Check sheet for the modelled part. Datum: model origin and axes. Units: mm. A direction names the side the tool comes from. Give positions to 0.01 mm unless a question says otherwise; leave off trailing zeros. Loops run counter-clockwise (first coordinate to the right, second up) from the corner with the lowest first, then second, coordinate; pieces in that order, holes last. Notation, with made-up numbers: M 7,20.5 L 44,20.5 A12 cw 44,35.5 Z; hole C 17,82 d4. An arc over 180 degrees is marked long. Use one line per item in the form item = value.
from build123d import *

# Parameters (mm, degrees)
SKETCH2_W           = 82.55
SKETCH2_H           = 38.1
BOSS_EXTRUDE1_DEPTH = 2.54
SKETCH3_W           = 71.12
SKETCH3_H           = 25.4
BOSS_EXTRUDE2_DEPTH = 5.08
SKETCH4_W           = 68.58
SKETCH4_H           = 22.86
CUT_EXTRUDE1_DEPTH  = 1.27
CUT_EXTRUDE1_DRAFT  = -18
SKETCH5_R           = 2.54
CUT_EXTRUDE2_DEPTH  = 2.54


with BuildPart() as part:
    # Sketch2 → Boss-Extrude1 (new body)
    with BuildSketch(Plane(origin=(0, 0, 0), x_dir=(1, 0, 0), z_dir=(0, 1, 0))):
        Rectangle(SKETCH2_W, SKETCH2_H)
    extrude(amount=BOSS_EXTRUDE1_DEPTH)

    # Sketch3 → Boss-Extrude2 (add)
    with BuildSketch(Plane(origin=(0, 2.54, 0), x_dir=(1, 0, 0), z_dir=(0, 1, 0))):
        Rectangle(SKETCH3_W, SKETCH3_H)
    extrude(amount=BOSS_EXTRUDE2_DEPTH)


with BuildPart() as cut_extrude1_tool:
    # Sketch4 → Cut-Extrude1 (with draft: the straight prism first)
    with BuildSketch(Plane(origin=(0, 7.62, 0), x_dir=(1, 0, 0), z_dir=(0, 1, 0))):
        Rectangle(SKETCH4_W, SKETCH4_H)
    extrude(amount=-CUT_EXTRUDE1_DEPTH)
    # Cut-Extrude1: the draft: its side faces are tilted about the plane it starts from
    cut_extrude1_sides = [cut_extrude1_tool.faces().sort_by_distance(p)[0] for p in [
        (-34.29, 6.985, 0),
        (0, 6.985, 11.43),
        (34.29, 6.985, 0),
        (0, 6.985, -11.43),
    ]]
    draft(cut_extrude1_sides, Plane(origin=(0, 7.62, 0), x_dir=(1, 0, 0), z_dir=(0, 1, 0)), CUT_EXTRUDE1_DRAFT)


with BuildPart() as part_1:
    add(part.part)

    # Cut-Extrude1: cut by cut_extrude1_tool
    add(cut_extrude1_tool.part, mode=Mode.SUBTRACT)

    # Sketch5 → Cut-Extrude2 (cut)
    with BuildSketch(Plane(origin=(0, 2.54, 0), x_dir=(1, 0, 0), z_dir=(0, 1, 0))):
        with Locations(Location((-37.465, 15.875, 0), (0, 0, 270))):
            Circle(SKETCH5_R)
        with Locations(Location((-37.465, -15.875, 0), (0, 0, 270))):
            Circle(SKETCH5_R)
        with Locations(Location((37.465, -15.875, 0), (0, 0, 270))):
            Circle(SKETCH5_R)
        with Locations(Location((37.465, 15.875, 0), (0, 0, 270))):
            Circle(SKETCH5_R)
    extrude(amount=-CUT_EXTRUDE2_DEPTH, mode=Mode.SUBTRACT)


solid = part_1.part
1) Section check C-C (z = 17.5). Record the cut outline in (x, y) (3 decimals), then the cut area to 3 significant figures.
Evaluation:
outline = M -41.275,0 L -39.417,0 L -39.417,2.54 L -41.275,2.54 Z; M -35.513,0 L 35.513,0 L 35.513,2.54 L -35.513,2.54 Z; M 39.417,0 L 41.275,0 L 41.275,2.54 L 39.417,2.54 Z
area = 190 mm^2
2) Section check B-B (x = 29). Record the cut outline in (y, z).
Evaluation:
outline = M 0,-19.05 L 2.54,-19.05 L 2.54,-12.7 L 7.62,-12.7 L 7.62,-11.43 L 6.35,-11.02 L 6.35,11.02 L 7.62,11.43 L 7.62,12.7 L 2.54,12.7 L 2.54,19.05 L 0,19.05 Z
3) Section check A-A (z = -1). Record the cut outline in (x, y) (3 decimals).
Evaluation:
outline = M -41.275,0 L 41.275,0 L 41.275,2.54 L 35.56,2.54 L 35.56,7.62 L 34.29,7.62 L 33.877,6.35 L -33.877,6.35 L -34.29,7.62 L -35.56,7.62 L -35.56,2.54 L -41.275,2.54 Z
4) Set-up check for faces 4 (the face through (0, 5, 12.7)), 5 (the face through (0, 6.35, 0)), 6 (the face through (0, 5, -12.7)), 7 (the face through (-35.56, 5, 0)), 8 (the face through (35.56, 5, 0)): record each of +Z, -Z, +X, -X, +Y, -Y from which the full face is reachable in a straight line by a thin tool's end or side.
Evaluation:
face_4 = +Z, +X, -X, +Y
face_5 = +Y
face_6 = -Z, +X, -X, +Y
face_7 = +Z, -Z, -X, +Y
face_8 = +Z, -Z, +X, +Y
5) Section check D-D (y = 3.5). Record the cut outline in (x, z).
Evaluation:
outline = M -35.56,-12.7 L 35.56,-12.7 L 35.56,12.7 L -35.56,12.7 Z
6) Release check for a two-part mould opening along Z. For faces 1 (the face through (35.212, 1.288, -14.703)), 2 (the face through (-1, 1, -19.05)), 3 (the face through (-1, 2.54, -13)) record: pulls with the +Z half, pulls with the -Z half, needs draft (parallel to the pull), parting line crosses it, or undercut.
Evaluation:
face_1 = undercut
face_2 = pulls with the -Z half
face_3 = needs draft
7) Depth check by flat-ended pin: pin 1 Ø4.5 at (x, z) = (-37.465, -15.875) entering from +Y; pin 2 Ø4 at (x, z) = (-2, 4.5) entering from +Y; pin 3 Ø4 at (x, y) = (10.5, 4) entering from +Z; pin 4 Ø4 at (y, z) = (5.5, 8.5) entering from +X. Enter the tip coordinate at first touch or a pass-through.
Evaluation:
pin_1 = through
pin_2 = 6.35
pin_3 = 19.05
pin_4 = 35.56
8) Scan lines: line 1 (X direction, y = 1.5, z = -14) (3 decimals); line 2 (X direction, y = 2.75, z = -6.5); line 3 (Z direction, x = -8, y = 6). Record each from-to range of solid material in increasing order.
Evaluation:
line_1 = -41.275 to -39.178, -35.752 to 35.752, 39.178 to 41.275
line_2 = -35.56 to 35.56
line_3 = -12.7 to 12.7
